```python
from build123d import *

# Parameters (mm, degrees)
SKETCH1_R           = 8.5
SKETCH1_R_2         = 1.7
BOSS_EXTRUDE1_DEPTH = 32.2
SKETCH2_R           = 2.6
CUT_EXTRUDE1_DEPTH  = 2.2


with BuildPart() as part:
    # Sketch1 → Boss-Extrude1 (new body)
    with BuildSketch(Plane(origin=(0, 0, 0), x_dir=(1, 0, 0), z_dir=(0, 1, 0))):
        Circle(SKETCH1_R)
        with Locations((0, 5)):
            Circle(SKETCH1_R_2, mode=Mode.SUBTRACT)
        with Locations((4.330127019, -2.5)):
            Circle(SKETCH1_R_2, mode=Mode.SUBTRACT)
        with Locations((-4.330127019, -2.5)):
            Circle(SKETCH1_R_2, mode=Mode.SUBTRACT)
    extrude(amount=BOSS_EXTRUDE1_DEPTH)

    # Sketch2 → Cut-Extrude1 (cut)
    with BuildSketch(Plane(origin=(0, 32.2, 0), x_dir=(1, 0, 0), z_dir=(0, 1, 0))):
        with Locations((0, 5)):
            Circle(SKETCH2_R)
        with Locations((4.330127019, -2.5)):
            Circle(SKETCH2_R)
        with Locations((-4.330127019, -2.5)):
            Circle(SKETCH2_R)
    extrude(amount=-CUT_EXTRUDE1_DEPTH, mode=Mode.SUBTRACT)


solid = part.part
```
Geometry: final body of the model. Coordinates: model frame, mm. A direction names the side the tool comes from. Coordinates: 2 decimals unless noted, no trailing zeros. Order: outer loops, then holes, each group sorted by start corner. A loop starts at its lowest first (then second) coordinate and runs counter-clockwise, first axis right, second up. Notation, with made-up numbers: (-35.5, 22) - (-20.5, 22) arc R21 cw to (-20.5, 58) - close; hole circle Ø3 at (63.25, -4.75). An arc over 180 degrees is marked (long way). Return JSON: item names as keys, results as strings. Group by question number.
1. Set-up query: faces 4 (the face through (2.63, 14.79, 2.43)), 5 (the face through (-0.338, 31.115, -7.578)). Return all of +Z, -Z, +X, -X, +Y, -Y with unobstructed straight access to the full face (end or side cutting, diameter ignored); none if empty.
2. Cut plane C-C (z = 2.5). Output: boundary loops of the cut face in (x, y), plus the area to 3 significant figures.
3. Material intervals for line 1 along Z through (x, y) = (0, 20.5); line 2 along X through (y, z) = (17.5, 2.5); line 3 along X through (y, z) = (31.35, 2.5), sorted ascending. Write a range as [from, to].
4. Cut plane A-A (x = 0). Output: boundary loops of the cut face in (y, z), plus the area to 3 significant figures.
5. Cut plane D-D (y = 12.5). Output: boundary loops of the cut face in (x, z).
6. Pin query (flat end, axial travel): pin 1 (1.6 mm diameter, centred on x = -3.5, z = 1.5, fed in from +Y); pin 2 (3 mm diameter, centred on x = 0, z = -5, fed in from +Y); pin 3 (1.5 mm diameter, centred on y = 22, z = 6.5, fed in from +X). Return the tip coordinate at first contact, or that it passes through.
7. Pull-direction query (Z, two-part tool) for faces 1 (the face through (0, 32.2, 0)), 2 (the face through (4.57, 15.875, -7.167)), 3 (the face through (-0.37, 14.79, -3.34)); classes: pulls with the +Z half, pulls with the -Z half, needs draft (parallel to the pull), parting line crosses it, or undercut.
8. Cut plane B-B (z = -3.75). Output: boundary loops of the cut face in (x, y).
Resolved:
{
 "1": {"face 4": "+Y, -Y", "face 5": "+Y"},
 "2": {"outline": "(-8.12, 0) - (-6.03, 0) - (-6.03, 30) - (-6.93, 30) - (-6.93, 32.2) - (-8.12, 32.2) - close; (-2.63, 0) - (2.63, 0) - (2.63, 30) - (1.73, 30) - (1.73, 32.2) - (-1.73, 32.2) - (-1.73, 30) - (-2.63, 30) - close; (6.03, 0) - (8.12, 0) - (8.12, 32.2) - (6.93, 32.2) - (6.93, 30) - (6.03, 30) - close", "area": "296 mm²"},
 "3": {"line 1": "z = [-8.5, -6.7], [-3.3, 8.5]", "line 2": "x = [-8.12, -6.03], [-2.63, 2.63], [6.03, 8.12]", "line 3": "x = [-8.12, -6.93], [-1.73, 1.73], [6.93, 8.12]"},
 "4": {"outline": "(0, -8.5) - (32.2, -8.5) - (32.2, -7.6) - (30, -7.6) - (30, -6.7) - (0, -6.7) - close; (0, -3.3) - (30, -3.3) - (30, -2.4) - (32.2, -2.4) - (32.2, 8.5) - (0, 8.5) - close", "area": "434 mm²"},
 "5": {"outline": "circle Ø17 at (0, 0); hole circle Ø3.4 at (-4.33, 2.5); hole circle Ø3.4 at (0, -5); hole circle Ø3.4 at (4.33, 2.5)"},
 "6": {"pin 1": "stops at y = 30", "pin 2": "passes through", "pin 3": "stops at x = 6.26"},
 "7": {"face 1": "needs draft", "face 2": "parting line crosses it", "face 3": "undercut"},
 "8": {"outline": "(-7.63, 0) - (-1.15, 0) - (-1.15, 30) - (-2.28, 30) - (-2.28, 32.2) - (-7.63, 32.2) - close; (1.15, 0) - (7.63, 0) - (7.63, 32.2) - (2.28, 32.2) - (2.28, 30) - (1.15, 30) - close"}
}
